Check sheet for the modelled part. Datum: model origin and axes. Units: mm. Round coordinates to 2 decimals unless told otherwise and drop trailing zeros. Write each loop counter-clockwise with the first axis right and the second up, starting at its lowest first coordinate (ties: lowest second). Pieces come first, ordered by that corner, then holes. Notation, with made-up numbers: (84, 22) - (139, 22) arc R14 ccw to (139, 36) - close; hole circle Ø3 at (66, 20). An arc over 180 degrees is marked (long way). Answer as a JSON object with one key per item and string values. Group by question number.
Item 1: Sectioned sample at B-B on x = 20.32. Record the boundary of the cut face in (y, z), plus the area to 3 significant figures.
Item 2: Thickness scan on line 1 (Z direction, x = 45.72, y = 4.45); line 2 (Z direction, x = 45.72, y = 2.8); line 3 (X direction, y = 5.4, z = -82.55). Record the ranges inside material, lowest first.
Item 3: Gauge pin test, flat ends, axial feed: P1, Ø8, axis at x = 69.5, z = -26, coming from the -Y side; P2, Ø6, axis at x = 45.72, z = -82.55, coming from the -Y side. Record the tip position at first contact, or that the pin passes through.
Item 4: Sectioned sample at D-D on z = -133.35. Record the boundary of the cut face in (x, y), plus the area to 3 significant figures.
Item 5: Sectioned sample at C-C on x = 45.72. Record the boundary of the cut face in (y, z), plus the area to 3 significant figures.
Item 6: Sectioned sample at A-A on z = -25.4. Record the boundary of the cut face in (x, y), plus the area to 3 significant figures.
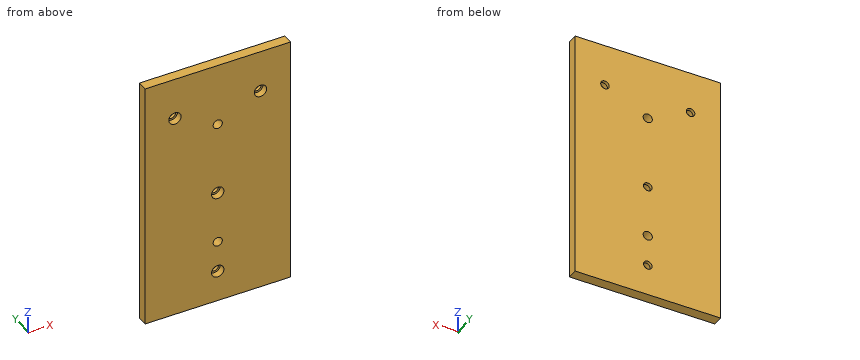
```python
from build123d import *

# Parameters (mm, degrees)
SKETCH2_W               = 88.9
SKETCH2_H               = 152.4
BOSS_EXTRUDE1_DEPTH     = 5.9944
SKETCH4_R               = 2.7305
CUT_EXTRUDE2_DEPTH      = 1
CUT_EXTRUDE2_DEPTH_BACK = 6.9944
SKETCH7_W               = 2.54
SKETCH7_H               = 152.4
CUT_EXTRUDE3_DEPTH      = 1
CUT_EXTRUDE3_DEPTH_BACK = 6.9944
SKETCH8_R               = 2.54
CUT_EXTRUDE4_DEPTH      = 1
CUT_EXTRUDE4_DEPTH_BACK = 6.9944
SKETCH9_R               = 3.683
CUT_EXTRUDE5_DEPTH      = 4.064


with BuildPart() as part:
    # Sketch2 → Boss-Extrude1 (new body)
    with BuildSketch(Plane(origin=(0, 0, 0), x_dir=(1, 0, 0), z_dir=(0, 1, 0))):
        with Locations((44.45, 76.2)):
            Rectangle(SKETCH2_W, SKETCH2_H)
    extrude(amount=BOSS_EXTRUDE1_DEPTH)

    # Sketch4 → Cut-Extrude2 (cut, two sides)
    with BuildSketch(Plane(origin=(0, 5.9944, 0), x_dir=(1, 0, 0), z_dir=(0, 1, 0))) as cut_extrude2_sk:
        with Locations((45.72, 114.3)):
            Circle(SKETCH4_R)
        with Locations((45.72, 38.1)):
            Circle(SKETCH4_R)
    extrude(amount=CUT_EXTRUDE2_DEPTH, mode=Mode.SUBTRACT)
    extrude(cut_extrude2_sk.sketch, amount=-CUT_EXTRUDE2_DEPTH_BACK, mode=Mode.SUBTRACT)

    # Sketch7 → Cut-Extrude3 (cut, two sides)
    with BuildSketch(Plane(origin=(0, 5.9944, 0), x_dir=(1, 0, 0), z_dir=(0, 1, 0))) as cut_extrude3_sk:
        with Locations((1.27, 76.2)):
            Rectangle(SKETCH7_W, SKETCH7_H)
    extrude(amount=CUT_EXTRUDE3_DEPTH, mode=Mode.SUBTRACT)
    extrude(cut_extrude3_sk.sketch, amount=-CUT_EXTRUDE3_DEPTH_BACK, mode=Mode.SUBTRACT)

    # Sketch8 → Cut-Extrude4 (cut, two sides)
    with BuildSketch(Plane(origin=(0, 5.9944, 0), x_dir=(1, 0, 0), z_dir=(0, 1, 0))) as cut_extrude4_sk:
        with Locations((20.32, 25.4)):
            Circle(SKETCH8_R)
        with Locations((71.12, 25.4)):
            Circle(SKETCH8_R)
        with Locations((45.72, 82.55)):
            Circle(SKETCH8_R)
        with Locations((45.72, 133.35)):
            Circle(SKETCH8_R)
    extrude(amount=CUT_EXTRUDE4_DEPTH, mode=Mode.SUBTRACT)
    extrude(cut_extrude4_sk.sketch, amount=-CUT_EXTRUDE4_DEPTH_BACK, mode=Mode.SUBTRACT)

    # Sketch9 → Cut-Extrude5 (cut)
    with BuildSketch(Plane.XZ):
        with Locations((20.32, -25.4)):
            Circle(SKETCH9_R)
        with Locations((71.12, -25.4)):
            Circle(SKETCH9_R)
        with Locations((45.72, -82.55)):
            Circle(SKETCH9_R)
        with Locations((45.72, -133.35)):
            Circle(SKETCH9_R)
    extrude(amount=-CUT_EXTRUDE5_DEPTH, mode=Mode.SUBTRACT)


solid = part.part
```
Completed:
{
 "1": {"outline": "(0, -152.4) - (5.99, -152.4) - (5.99, -27.94) - (4.06, -27.94) - (4.06, -29.08) - (0, -29.08) - close; (0, -21.72) - (4.06, -21.72) - (4.06, -22.86) - (5.99, -22.86) - (5.99, 0) - (0, 0) - close", "area": "874 mm²"},
 "2": {"line 1": "-152.4 to -135.89, -130.81 to -117.03, -111.57 to -85.09, -80.01 to -40.83, -35.37 to 0", "line 2": "-152.4 to -137.03, -129.67 to -117.03, -111.57 to -86.23, -78.87 to -40.83, -35.37 to 0", "line 3": "2.54 to 43.18, 48.26 to 88.9"},
 "3": {"P1": "y = 0", "P2": "y = 4.06"},
 "4": {"outline": "(2.54, 0) - (42.04, 0) - (42.04, 4.06) - (43.18, 4.06) - (43.18, 5.99) - (2.54, 5.99) - close; (48.26, 4.06) - (49.4, 4.06) - (49.4, 0) - (88.9, 0) - (88.9, 5.99) - (48.26, 5.99) - close", "area": "478 mm²"},
 "5": {"outline": "(0, -152.4) - (5.99, -152.4) - (5.99, -135.89) - (4.06, -135.89) - (4.06, -137.03) - (0, -137.03) - close; (0, -129.67) - (4.06, -129.67) - (4.06, -130.81) - (5.99, -130.81) - (5.99, -117.03) - (0, -117.03) - close; (0, -111.57) - (5.99, -111.57) - (5.99, -85.09) - (4.06, -85.09) - (4.06, -86.23) - (0, -86.23) - close; (0, -78.87) - (4.06, -78.87) - (4.06, -80.01) - (5.99, -80.01) - (5.99, -40.83) - (0, -40.83) - close; (0, -35.37) - (5.99, -35.37) - (5.99, 0) - (0, 0) - close", "area": "769 mm²"},
 "6": {"outline": "(2.54, 0) - (16.64, 0) - (16.64, 4.06) - (17.78, 4.06) - (17.78, 5.99) - (2.54, 5.99) - close; (22.86, 4.06) - (24, 4.06) - (24, 0) - (67.44, 0) - (67.44, 4.06) - (68.58, 4.06) - (68.58, 5.99) - (22.86, 5.99) - close; (73.66, 4.06) - (74.8, 4.06) - (74.8, 0) - (88.9, 0) - (88.9, 5.99) - (73.66, 5.99) - close", "area": "438 mm²"}
}
